The drawing under review shows one solid part. Ordinate dimensions are in mm from its lowest x, y, z. Round coordinates to 2 decimals unless told otherwise and drop trailing zeros. Write each loop counter-clockwise with the first axis right and the second up, starting at its lowest first coordinate (ties: lowest second). Pieces come first, ordered by that corner, then holes. Notation, with made-up numbers: (67, -3.75) -> (92, -3.75) arc R17 ccw to (92, 29.25) -> close; hole circle Ø9 at (24, 63). An arc over 180 degrees is marked (long way). Answer in a Markdown table with one row per item.
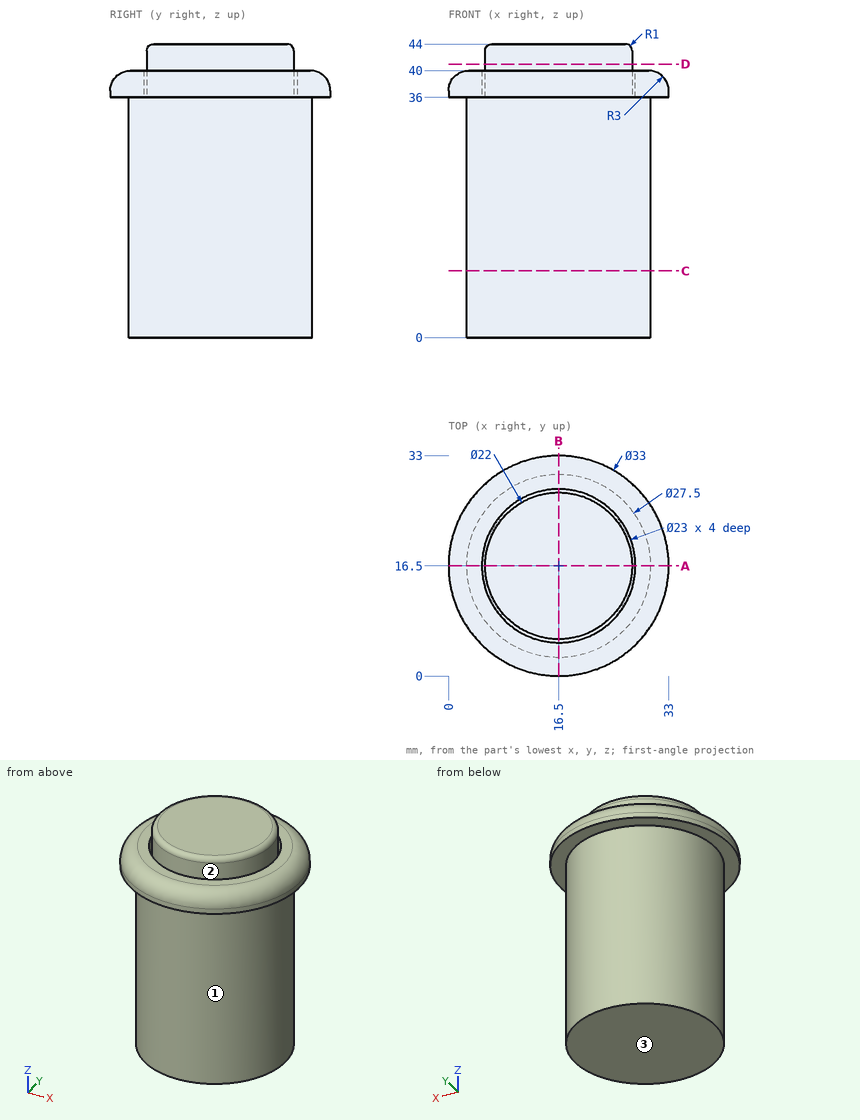
1) Clearance check with flat-ended pins moving along their axes: pin 1 Ø12 at (y, z) = (17.5, 14.5) entering from +X; pin 2 Ø3 at (x, z) = (24.5, 12.5) entering from +Y; pin 3 Ø6 at (x, z) = (9, 21) entering from -Y. State where each tip first meets the part, or that it passes through.
Solved:
| item | result |
|---|---|
| pin 1 | x = 30.25 |
| pin 2 | y = 28.62 |
| pin 3 | y = 3.51 |
2) Mouldability with a two-part tool opening along Y and no side actions: class the marked faces 1, 2 and 3 as pulls with the +Y half, pulls with the -Y half, needs draft (parallel to the pull), parting line crosses it, or undercut.
Solved:
| item | result |
|---|---|
| face 1 | parting line crosses it |
| face 2 | undercut |
| face 3 | needs draft |
3) Consider section C-C on z = 10. State the section outline as (x, y) points, then the cut area to 3 significant figures.
Solved:
| item | result |
|---|---|
| outline | circle Ø27.5 at (16.5, 16.5) |
| area | 594 mm² |
4) Consider section A-A on y = 16.5. State the section outline as (x, z) points.
Solved:
| item | result |
|---|---|
| outline | (0, 36) -> (2.75, 36) -> (2.75, 0) -> (30.25, 0) -> (30.25, 36) -> (33, 36) -> (33, 37) arc R3 ccw to (30, 40) -> (28, 40) -> (28, 36) -> (27.5, 36) -> (27.5, 43) arc R1 ccw to (26.5, 44) -> (6.5, 44) arc R1 ccw to (5.5, 43) -> (5.5, 36) -> (5, 36) -> (5, 40) -> (3, 40) arc R3 ccw to (0, 37) -> close |
5) For line 1 (Y direction, x = 16, z = 37); line 2 (Y direction, x = 16, z = 39); line 3 (X direction, y = 16, z = 38), list the stretches that pass through material, from the lowest coordinate up. Write a range as [from, to].
Solved:
| item | result |
|---|---|
| line 1 | [0.01, 5.01], [5.51, 27.49], [27.99, 32.99] |
| line 2 | [0.77, 5.01], [5.51, 27.49], [27.99, 32.23] |
| line 3 | [0.18, 5.01], [5.51, 27.49], [27.99, 32.82] |
6) Consider section D-D on z = 41. State the section outline as (x, y) points.
Solved:
| item | result |
|---|---|
| outline | circle Ø22 at (16.5, 16.5) |
